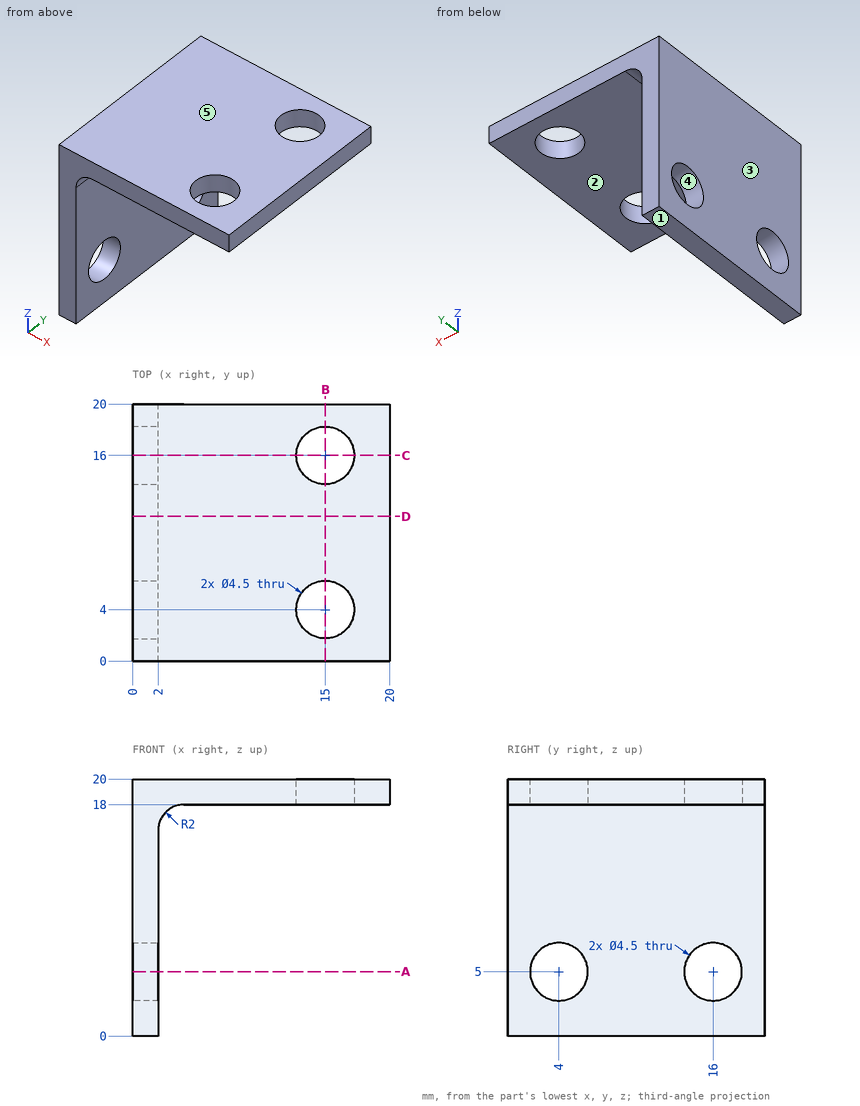
Here's the drawing with two shaded views (mm, measured from the low corner). I have some questions. A direction names the side the tool comes from. Round coordinates to 2 decimals unless told otherwise and drop trailing zeros. Order: outer loops, then holes, each group sorted by start corner. A loop starts at its lowest first (then second) coordinate and runs counter-clockwise, first axis right, second up. Notation, with made-up numbers: (63.5, 9.5) -> (71.5, 9.5) arc R30 cw to (71.5, 47.5) -> close; hole circle Ø9 at (50, 44.5). An arc over 180 degrees is marked (long way). Write each question's results on one line, items separated by ' | '. Start each with the question number.
Item 1: If we section it at A-A, the plane z = 5: Write out the boundary of the cut face in (x, y).
Item 2: Which directions (+Z, -Z, +X, -X, +Y, -Y) give clear straight access to the entire face, cutting with the end or side of a thin tool? Please do the marked faces 1 and 2.
Item 3: If we section it at B-B, the plane x = 15: Write out the boundary of the cut face in (y, z).
Item 4: If we section it at C-C, the plane y = 16: Write out the boundary of the cut face in (x, z), then the cut area to 3 significant figures.
Item 5: If we section it at D-D, the plane y = 11.25: Write out the boundary of the cut face in (x, z).
Item 6: Will these pins go through, and if not, where does the flat tip stop? pin 1 (4 mm diameter, centred on x = 15, y = 4, fed in from -Z); pin 2 (5 mm diameter, centred on x = 15, y = 16, fed in from -Z).
Item 7: Please list where these lines run through material, in increasing order: L1, parallel to Y at x = 1.25, z = 5; L2, parallel to X at y = 17.5, z = 11; L3, parallel to Z at x = 8.25, y = 1.5.
Item 8: Thinking about a two-plate mould opening in Z: for the marked faces 3, 4 and 5, which applies, +Z half, -Z half, draft (parallel to the pull), parting line (faces both ways), or undercut?
Results:
1) outline: (0, 0) -> (2, 0) -> (2, 1.75) -> (0, 1.75) -> close; (0, 6.25) -> (2, 6.25) -> (2, 13.75) -> (0, 13.75) -> close; (0, 18.25) -> (2, 18.25) -> (2, 20) -> (0, 20) -> close
2) face 1: -Z, +X, -X, +Y, -Y | face 2: -Z, +X, +Y, -Y
3) outline: (0, 18) -> (1.75, 18) -> (1.75, 20) -> (0, 20) -> close; (6.25, 18) -> (13.75, 18) -> (13.75, 20) -> (6.25, 20) -> close; (18.25, 18) -> (20, 18) -> (20, 20) -> (18.25, 20) -> close
4) outline: (0, 0) -> (2, 0) -> (2, 2.75) -> (0, 2.75) -> close; (0, 7.25) -> (2, 7.25) -> (2, 16) arc R2 cw to (4, 18) -> (12.75, 18) -> (12.75, 20) -> (0, 20) -> close; (17.25, 18) -> (20, 18) -> (20, 20) -> (17.25, 20) -> close | area: 58.9 mm2
5) outline: (0, 0) -> (2, 0) -> (2, 16) arc R2 cw to (4, 18) -> (20, 18) -> (20, 20) -> (0, 20) -> close
6) pin 1: passes through | pin 2: stops at z = 18
7) L1: y = 0 to 1.75, 6.25 to 13.75, 18.25 to 20 | L2: x = 0 to 2 | L3: z = 18 to 20
8) face 3: draft | face 4: undercut | face 5: +Z half
